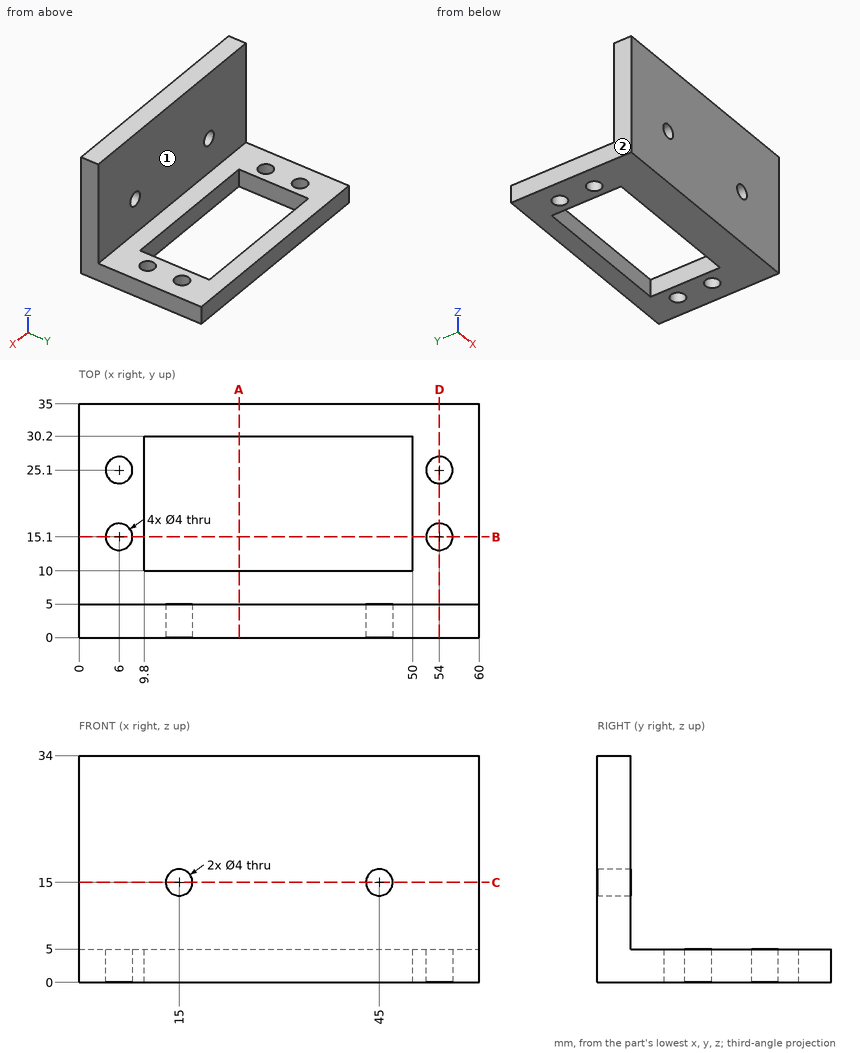
Design review of the part shown in the three views and the two pictorial views. Dimensions are in mm from the part's minimum x, y and z. A direction names the side the tool comes from. Round coordinates to 2 decimals unless told otherwise and drop trailing zeros. Loops run counter-clockwise (first coordinate to the right, second up) from the corner with the lowest first, then second, coordinate; pieces in that order, holes last. Notation, with made-up numbers: M 60.5,-24 L 111.5,-24 A35 ccw 111.5,9 Z; hole C -7.5,-5 d5. An arc over 180 degrees is marked long. Answer as a JSON object with one key per item and string values.
Item 1: We need section A-A on x = 24. Give the boundary of the cut face in (y, z).
Answer sheet:
{"outline": "M 0,0 L 10,0 L 10,5 L 5,5 L 5,34 L 0,34 Z; M 30.2,0 L 35,0 L 35,5 L 30.2,5 Z"}
Item 2: Clearance check with flat-ended pins moving along their axes: P1, Ø6.5, axis at x = 6, y = 25.1, coming from the -Z side; P2, Ø2, axis at x = 30.5, z = 29, coming from the +Y side; P3, Ø3, axis at x = 54, y = 15.1, coming from the -Z side; P4, Ø6.5, axis at x = 54, y = 25.1, coming from the +Z side. State where each tip first meets the part, or that it passes through.
Answer sheet:
{"P1": "stops at z = 0", "P2": "stops at y = 5", "P3": "passes through", "P4": "stops at z = 5"}
Item 3: Machinability: for the marked faces 1 and 2, which of the approach directions +Z, -Z, +X, -X, +Y, -Y give a long, thin tool a straight path to every point of the face, cutting with its end or side? Answer none if there is none.
Answer sheet:
{"face 1": "+Z, +X, -X, +Y", "face 2": "+Z, -Z, -X, +Y, -Y"}
Item 4: We need section B-B on y = 15.1. Give the boundary of the cut face in (x, z).
Answer sheet:
{"outline": "M 0,0 L 4,0 L 4,5 L 0,5 Z; M 8,0 L 9.8,0 L 9.8,5 L 8,5 Z; M 50,0 L 52,0 L 52,5 L 50,5 Z; M 56,0 L 60,0 L 60,5 L 56,5 Z"}
Item 5: We need section D-D on x = 54. Give the boundary of the cut face in (y, z), and give its area (3 significant figures).
Answer sheet:
{"outline": "M 0,0 L 13.1,0 L 13.1,5 L 5,5 L 5,34 L 0,34 Z; M 17.1,0 L 23.1,0 L 23.1,5 L 17.1,5 Z; M 27.1,0 L 35,0 L 35,5 L 27.1,5 Z", "area": "280 mm^2"}
Item 6: We need section C-C on z = 15. Give the boundary of the cut face in (x, y).
Answer sheet:
{"outline": "M 0,0 L 13,0 L 13,5 L 0,5 Z; M 17,0 L 43,0 L 43,5 L 17,5 Z; M 47,0 L 60,0 L 60,5 L 47,5 Z"}
Item 7: Wall thickness on L1, parallel to Y at x = 6, z = 1.65; L2, parallel to X at y = 3.05, z = 15; L3, parallel to Z at x = 15, y = 1.15: over which ranges is each line inside the solid? List them lowest first. Write a range as from..to.
Answer sheet:
{"L1": "y = 0..13.1, 17.1..23.1, 27.1..35", "L2": "x = 0..13, 17..43, 47..60", "L3": "z = 0..13, 17..34"}
